```python
from build123d import *

# Parameters (mm, degrees)
BOSS_EXTRUDE1_DEPTH = 45
BOSS_EXTRUDE2_START = -10
BOSS_EXTRUDE2_DEPTH = 70
SKETCH3_R           = 25
SKETCH3_R_2         = 15
BOSS_EXTRUDE3_DEPTH = 30


with BuildPart() as part:
    # Sketch1 → Boss-Extrude1 (new, symmetric)
    with BuildSketch(Plane(origin=(0, 0, 0), x_dir=(0, 0, -1), z_dir=(1, 0, 0))):
        Polygon((-20.642857143, -6.642857143), (-30.642857143, -6.642857143), (-30.642857143, 8.357142857), (19.357142857, 8.357142857), (19.357142857, -6.642857143), (9.357142857, -6.642857143), (9.357142857, -1.642857143), (-20.642857143, -1.642857143), align=None)
    extrude(amount=BOSS_EXTRUDE1_DEPTH, both=True)

    # Sketch2 → Boss-Extrude2 (add)
    with BuildSketch(Plane(origin=(45, 0, 0), x_dir=(0, 0, -1), z_dir=(1, 0, 0)).offset(BOSS_EXTRUDE2_START)):
        with BuildLine():
            Line((19.357142857, 8.357142857), (19.357142857, 38.357142857))
            ThreePointArc((19.357142857, 38.357142857), (20.821608951, 41.892676763), (24.357142857, 43.357142857))
            Line((24.357142857, 43.357142857), (94.357142857, 43.357142857))
            ThreePointArc((94.357142857, 43.357142857), (97.892676763, 41.892676763), (99.357142857, 38.357142857))
            Line((99.357142857, 38.357142857), (99.357142857, 8.357142857))
            Line((99.357142857, 8.357142857), (109.357142857, 8.357142857))
            Line((109.357142857, 8.357142857), (109.357142857, 38.357142857))
            ThreePointArc((109.357142857, 38.357142857), (104.963744575, 48.963744575), (94.357142857, 53.357142857))
            Line((94.357142857, 53.357142857), (24.357142857, 53.357142857))
            ThreePointArc((24.357142857, 53.357142857), (13.750541139, 48.963744575), (9.357142857, 38.357142857))
            Line((9.357142857, 38.357142857), (9.357142857, 8.357142857))
            Line((9.357142857, 8.357142857), (19.357142857, 8.357142857))
        make_face()
    extrude(amount=-BOSS_EXTRUDE2_DEPTH)

    # Sketch3 → Boss-Extrude3 (add)
    with BuildSketch(Plane(origin=(0, 53.357142857, 0), x_dir=(1, 0, 0), z_dir=(0, 1, 0))):
        with Locations(Location((0, 59.357142857, 0), (0, 0, 270))):
            Circle(SKETCH3_R)
        with Locations(Location((0, 59.357142857, 0), (0, 0, 270))):
            Circle(SKETCH3_R_2, mode=Mode.SUBTRACT)
    extrude(amount=BOSS_EXTRUDE3_DEPTH)


solid = part.part
```
Work out the finished part from the listing and answer in its coordinate system (mm). A direction names the side the tool comes from. Give positions to 0.01 mm unless a question says otherwise; leave off trailing zeros. Loops run counter-clockwise (first coordinate to the right, second up) from the corner with the lowest first, then second, coordinate; pieces in that order, holes last. Notation, with made-up numbers: M 24.25,40.5 L 52.25,40.5 A15 cw 52.25,49.5 Z; hole C -5,2.5 d7. An arc over 180 degrees is marked long. One line per item, written item: value. Start each with the question number.
1. Determine the mould class of faces 5 (the face through (0, 23, -109.357)), 6 (the face through (0, 53.357, -60)), 7 (the face through (0.49, 41.931, -97.854)), 8 (the face through (45, 3, 5)) for opening direction Z: released by +Z, released by -Z, zero draft, split by the parting line, or undercut.
2. Find section A-A (y = 24.5). Give the vertices of the cut face in (x, z), and give its area (3 significant figures).
3. Find section C-C (z = -76.5). Give the vertices of the cut face in (x, y).
4. Find section B-B (x = 38.5). Give the vertices of the cut face in (y, z).
5. Each of these flat-tipped pins is pushed along its axis until it touches: P1, Ø5, axis at x = -16.5, y = 22.5, coming from the +Z side; P2, Ø22.5, axis at x = 5.5, y = 6, coming from the -Z side; P3, Ø24, axis at x = 0, z = -59.36, coming from the +Y side; P4, Ø15, axis at x = -21.5, z = -1.5, coming from the +Y side. Where does it stop, or does it pass through?
6. Which of the six approach directions +Z, -Z, +X, -X, +Y, -Y give full straight-line access (tool end or side, diameter ignored) to faces 1 (the face through (1, -6.643, 26)), 2 (the face through (0, 8.357, -104)), 3 (the face through (1, 16, -19.357)), 4 (the face through (-15.21, 68.15, -79.2))?
7. Find section D-D (y = 74). Give the vertices of the cut face in (x, z).
8. Find the intervals of material crossed by probe 1 along Z at (x, y) = (18, 9); probe 2 along Y at (x, z) = (-28, 0); probe 3 along Y at (x, z) = (3, -90), in increasing order.
Reported:
1. face 5: released by -Z
1. face 6: undercut
1. face 7: undercut
1. face 8: zero draft
2. outline: M -35,-109.36 L 35,-109.36 L 35,-99.36 L -35,-99.36 Z; M -35,-19.36 L 35,-19.36 L 35,-9.36 L -35,-9.36 Z
2. area: 1,400 mm²
3. outline: M -35,43.36 L 35,43.36 L 35,53.36 L 18.2,53.36 L 18.2,83.36 L -18.2,83.36 L -18.2,53.36 L -35,53.36 Z
4. outline: M -6.64,-19.36 L 8.36,-19.36 L 8.36,30.64 L -6.64,30.64 L -6.64,20.64 L -1.64,20.64 L -1.64,-9.36 L -6.64,-9.36 Z
5. P1: stops at z = -9.36
5. P2: stops at z = -109.36
5. P3: stops at y = 53.36
5. P4: stops at y = 8.36
6. face 1: +Z, -Z, +X, -X, -Y
6. face 2: -Z, +X, -X, -Y
6. face 3: +X, -X, -Y
6. face 4: +Y
7. outline: C 0,-59.36 d50; hole C 0,-59.36 d30
8. probe 1: z = -109.36 to -99.36, -19.36 to -9.36
8. probe 2: y = -1.64 to 8.36
8. probe 3: y = 43.36 to 53.36
